Autodesk Inventor part; units mm, degrees
ref_plane "YZ Plane" through (0, 0, 0) normal (1, 0, 0) x (0, 1, 0)
ref_plane "XZ Plane" through (0, 0, 0) normal (0, 1, 0) x (-1, 0, 0)
ref_plane "XY Plane" through (0, 0, 0) normal (0, 0, 1) x (1, 0, 0)
sketch "スケッチ1" plane through (0, 0, 0) normal (1, 0, 0) x (0, 1, 0)
  line L0 (0, 0) -> (38, 0)
  line L1 (38, 0) -> (38, -60)
  line L2 (38, -60) -> (0, -60)
  line L3 (0, -60) -> (0, 0)
  dimension "d0" = 60
  dimension "d1" = 38
extrude "押し出し1" add sketch "スケッチ1" along normal blind 41
sketch "スケッチ4" plane through (0, 0, 0) normal (-1, 0, 0) x (0, 0, 1)
  line L0 (0, 0) -> (-60, 0)
  line L1 (0, 38) -> (0, 0)
  point P0 (-29, 34)
  point P1 (-9, 34)
  point P2 (-9, 4)
  point P3 (-29, 4)
  dimension "d4" = 20
  dimension "d5" = 30
  dimension "d7" = 9
  dimension "d15" = 4
hole "穴1" at (0, 34, -29) at (0, 34, -9) at (0, 4, -9) at (0, 4, -29) direction (1, 0, 0) diameter 2.459 depth 8.8 tip angle 118
For this review, take the finished solid that the model builds, in its own axes (mm). A direction names the side the tool comes from. Coordinates: 2 decimals unless noted, no trailing zeros. Put each result on its own line as item: value.
1. For pin 1 (6 mm diameter, centred on y = 5, z = -30.5, fed in from -X), flat-tipped, find the tip position at first contact; note if it passes through.
Values found:
pin 1: x = 0
2. Machinability: for faces 4 (the cylindrical face through (4.46, 32.78, -29.16)), 5 (the flat face through (20, 38, -30)), which of the approach directions +Z, -Z, +X, -X, +Y, -Y give a long, thin tool a straight path to every point of the face, cutting with its end or side? Answer none if there is none.
Values found:
face 4: -X
face 5: +Z, -Z, +X, -X, +Y
3. Mouldability with a two-part tool opening along Z and no side actions: class faces 1 (the flat face through (20, 19, 0)), 2 (the flat face through (41, 19, -30)), 3 (the cylindrical face through (4.46, 32.78, -9.16)) as released by +Z, released by -Z, zero draft, split by the parting line, or undercut.
Values found:
face 1: released by +Z
face 2: zero draft
face 3: undercut
4. Wall thickness on probe 1 along Y at (x, z) = (5, -9); probe 2 along Z at (x, y) = (2.25, 4): over which ranges is each line inside the solid? List them lowest first.
Values found:
probe 1: 0 to 2.77, 5.23 to 32.77, 35.23 to 38
probe 2: -60 to -30.23, -27.77 to -10.23, -7.77 to 0
